Check sheet for the modelled part. Datum: model origin and axes. Units: mm. Face numbers are marked on the shaded views. A direction names the side the tool comes from. Give positions to 0.01 mm unless a question says otherwise; leave off trailing zeros. Loops run counter-clockwise (first coordinate to the right, second up) from the corner with the lowest first, then second, coordinate; pieces in that order, holes last. Notation, with made-up numbers: M 15,-14.5 L 61,-14.5 A26 ccw 61,4.5 Z; hole C -19.5,84.25 d10. An arc over 180 degrees is marked long. Put each result on its own line as item: value. Start each with the question number.
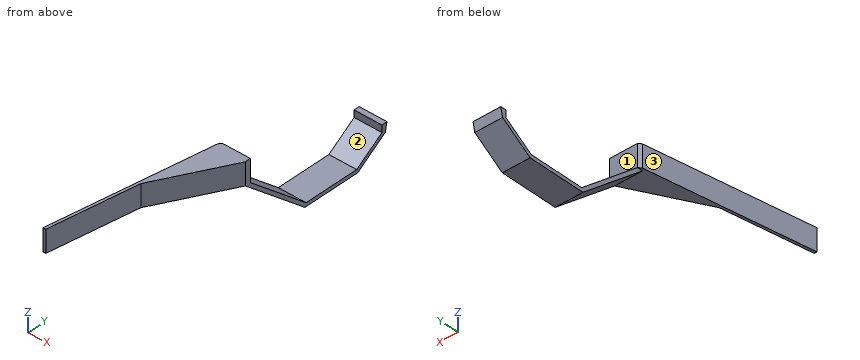
```python
from build123d import *

# Parameters (mm, degrees)
SKETCH_9_W          = 32
SKETCH_9_H          = 240
EXTRUDE_4_DEPTH     = 8
EXTRUDE_5_DEPTH     = 32
SKETCH_11_W         = 40
SKETCH_11_H         = 8
EXTRUDE_6_DEPTH     = 40
SKETCH_14_W         = 4
SKETCH_14_H         = 32
SKETCH_16_W         = 49.074899356
SKETCH_16_H         = 238.21753212
CUT_EXTRUDE_1_DEPTH = 40
EXTRUDE_7_DEPTH     = 32


with BuildPart() as part:
    # 草图9 → 凸台-拉伸4 (new body)
    with BuildSketch(Plane(origin=(0, 0, 0), x_dir=(0, 0, -1), z_dir=(1, 0, 0))):
        with Locations((0, 120)):
            Rectangle(SKETCH_9_W, SKETCH_9_H)
    extrude(amount=EXTRUDE_4_DEPTH)

    # 草图10 → 凸台-拉伸5 (add)
    with BuildSketch(Plane.XY.offset(16)):
        Polygon((40, 232), (8, 120), (8, 232), (8, 240), (40, 240), align=None)
    extrude(amount=-EXTRUDE_5_DEPTH)

    # 扫描8: sweep along a path in 草图12
    with BuildLine(Plane.ZY) as sweep_8_path:
        Line((-16, 240), (-90.839227599, 328))
        Line((-90.839227599, 328), (-90.839227599, 408))
        Line((-90.839227599, 408), (-63.750419078, 447.942286341))
        Line((-63.750419078, 447.942286341), (-53.704847623, 447.942286341))
    # 草图11 → 扫描8 (sweep)
    with BuildSketch(Plane(origin=(0, 0, -16), x_dir=(-1, 0, 0), z_dir=(0, 0, -1))):
        with Locations((-20, 236)):
            Rectangle(SKETCH_11_W, SKETCH_11_H)
    sweep(path=sweep_8_path.line, transition=Transition.RIGHT)

    # 草图13 → 凸台-拉伸6 (add)
    with BuildSketch(Plane.ZY):
        Polygon((-66.49773312, 453.125050648), (-53.704847623, 455.942286341), (-53.704847623, 447.942286341), (-63.750419078, 447.942286341), align=None)
    extrude(amount=-EXTRUDE_6_DEPTH)

    # 扫描9: sweep along a path in 草图15
    with BuildLine(Plane.XY.offset(16)) as sweep_9_path:
        Line((-36, 0), (0, 232))
        Line((0, 232), (40, 232))
    # 草图14 → 扫描9 (sweep)
    with BuildSketch(Plane.XZ):
        with Locations((-38, 0)):
            Rectangle(SKETCH_14_W, SKETCH_14_H)
    sweep(path=sweep_9_path.line, transition=Transition.RIGHT)

    # 草图16 → 切除-拉伸1 (cut)
    with BuildSketch(Plane.XY.offset(16)):
        with Locations((24.537449678, 112.89123394)):
            Rectangle(SKETCH_16_W, SKETCH_16_H)
    extrude(amount=-CUT_EXTRUDE_1_DEPTH, mode=Mode.SUBTRACT)

    # 草图17 → 凸台-拉伸7 (add)
    with BuildSketch(Plane.XY.offset(16)):
        Polygon((-3.386650681, 235.952695613), (0, 240), (40, 240), (40, 232), (-21.69332534, 117.976347807), align=None)
    extrude(amount=-EXTRUDE_7_DEPTH)


solid = part.part
```
Q1. Section check C-C, the plane y = 385.5. Record the cut outline in (x, z), then the cut area to 3 significant figures.
Q2. Section check A-A, the plane z = 1. Record the cut outline in (x, y), then the cut area to 3 significant figures.
Q3. Section check D-D, the plane x = 4.5. Record the cut outline in (y, z).
Q4. Access from +Z, -Z, +X, -X, +Y, -Y to the whole of each face (thin tool, end or side, straight path). Record for the marked faces 1, 2 and 3.
Q5. Thickness scan on line 1 along Z through (x, y) = (0.5, 212); line 2 along Y through (x, z) = (3.5, -79); line 3 along Y through (x, z) = (34, -71). Record the ranges inside material, lowest first. Write a range as [from, to].
Q6. Section check B-B, the plane x = 22. Record the cut outline in (y, z).
Q7. Depth check by flat-ended pin: P1, Ø20, axis at x = 19.5, y = 381, coming from the +Z side; P2, Ø11, axis at x = 22.5, z = -60.5, coming from the -Y side; P3, Ø9, axis at x = 28, y = 453, coming from the +Z side. Enter the tip coordinate at first touch or a pass-through.
Found:
1. outline: M 0,-96.02 L 40,-96.02 L 40,-90.84 L 0,-90.84 Z
1. area: 207 mm^2
2. outline: M -40,0 L -36,0 L -16.08,128.34 L 40,232 L 40,240 L 0,240 L -3.39,235.95 Z
2. area: 3,340 mm^2
3. outline: M 166.39,-16 L 232,-16 L 326.09,-96.02 L 409.59,-96.02 L 453.13,-66.5 L 455.94,-53.7 L 447.94,-53.7 L 447.94,-63.75 L 408,-90.84 L 328,-90.84 L 240,-16 L 240,16 L 166.39,16 Z
4. face 1: +Z, +X, -X, +Y
4. face 2: +Z, +X, -X
4. face 3: +Z, -Z, -X, +Y
5. line 1: z = [-16, 16]
5. line 2: y = [306.08, 314.08], [425.46, 434.69]
5. line 3: y = [296.67, 304.67], [437.25, 446.49]
6. outline: M 198.73,-16 L 232,-16 L 326.09,-96.02 L 409.59,-96.02 L 453.13,-66.5 L 455.94,-53.7 L 447.94,-53.7 L 447.94,-63.75 L 408,-90.84 L 328,-90.84 L 240,-16 L 240,16 L 198.73,16 Z
7. P1: stops at z = -90.84
7. P2: stops at y = 277.86
7. P3: stops at z = -53.7
